Autodesk Inventor part; units mm, degrees
ref_plane "YZ Plane" through (0, 0, 0) normal (1, 0, 0) x (0, 1, 0)
ref_plane "XZ Plane" through (0, 0, 0) normal (0, 1, 0) x (-1, 0, 0)
ref_plane "XY Plane" through (0, 0, 0) normal (0, 0, 1) x (1, 0, 0)
sketch "Sketch1" plane through (0, 0, 0) normal (0, 0, 1) x (1, 0, 0)
  line L0 (-12.5919, 2.2112) -> (12.8081, 2.2112)
  line L1 (12.8081, 2.2112) -> (12.8081, 8.9549)
  line L2 (12.8081, 8.9549) -> (8.7187, 5.3862)
  line L3 (8.7187, 5.3862) -> (-12.5919, 5.3862)
  line L4 (-12.5919, 5.3862) -> (-12.5919, 2.2112)
  dimension "d0" = 3.175
  dimension "d2" = 4.0894
  dimension "d3" = 6.7437
  dimension "d19" = 25.4
revolve "Revolution1" add sketch "Sketch1" angle 360 about axis through (-12.5919, 2.2112, 0) along (1, 0, 0)
thread "Thread1"
sketch "Sketch2" plane through (12.8081, 2.2112, 0) normal (1, 0, 0) x (0, 0, -1)
  circle A0 centre (0, 0) radius 6.7437
  line L0 (0, -2.2914) -> (-1.9844, -1.1457)
  line L1 (-1.9844, -1.1457) -> (-1.9844, 1.1457)
  line L2 (-1.9844, 1.1457) -> (0, 2.2914)
  line L3 (0, 2.2914) -> (1.9844, 1.1457)
  line L4 (1.9844, 1.1457) -> (1.9844, -1.1457)
  line L5 (1.9844, -1.1457) -> (0, -2.2914)
  dimension "d16" = 3.9688
extrude "Extrusion1" cut sketch "Sketch2" against normal blind 1.905 contours L0 L1 L2 L3 L4 L5
properties part number "HW-00074"
Input: part model. Units: mm. Frame: model coordinates. A direction names the side the tool comes from. Round coordinates to 2 decimals unless told otherwise and drop trailing zeros. Loops run counter-clockwise (first coordinate to the right, second up) from the corner with the lowest first, then second, coordinate; pieces in that order, holes last. Notation, with made-up numbers: M 15.5,-21 L 72.5,-21 A30 cw 72.5,17 Z; hole C 38.25,-31 d1. An arc over 180 degrees is marked long. Answer as CSV lines item,"result". Start each with the question number.
(1) First-contact query: pin 1 (2 mm diameter, centred on y = 2, z = 0.5, fed in from +X); pin 2 (8 mm diameter, centred on x = -0.5, y = 1, fed in from +Z) (3 decimals); pin 3 (2 mm diameter, centred on x = -4.5, y = 6, fed in from -Z). Flat tips, straight axial feed; report the tip coordinate or a pass-through.
(2) Section A-A, the plane x = -9.5. Output: boundary loops of the cut face in (y, z) (3 decimals), plus the area to 3 significant figures.
(3) Line query: line 1 (X direction, y = 1, z = 0.25); line 2 (Y direction, x = 11.75, z = -1.75); line 3 (X direction, y = -1, z = 2.25). Output: solid intervals per line, ascending. Write a range as [from, to].
(4) Draft query along Z for faces 3 (the cylindrical face through (-2.09, 5.24, -0.95)), 4 (the flat face through (11.869, 3.938, -0.978)), 5 (the flat face through (-12.592, 2, 0)). Return one class per face: released by +Z, released by -Z, zero draft, split by the parting line, or undercut.
(5) Reachability of faces 1 (the flat face through (12.808, 4, 2)), 2 (the flat face through (10.903, 2, 0)) from +Z, -Z, +X, -X, +Y, -Y: full face, straight path, thin tool, end or side. Return the list, or none.
Values found:
1,pin 1,"stops at x = 10.9"
1,pin 2,"stops at z = 3.175"
1,pin 3,"stops at z = -1.52"
2,outline,"C 2.211,0 d6.35"
2,area,"31.7 mm²"
3,line 1,"x = [-12.59, 10.9]"
3,line 2,"y = [-3.34, 0.93], [3.49, 7.76]"
3,line 3,"x = [9.57, 12.81]"
4,face 3,"split by the parting line"
4,face 4,"undercut"
4,face 5,"zero draft"
5,face 1,"+Z, -Z, +X, +Y, -Y"
5,face 2,"+X"
